from build123d import *

# Parameters (mm, degrees)
F1_DEPTH = 25
F2_R     = 1.5
F3_DEPTH = 1.5
F4_R     = 1.5
F5_DEPTH = 1.5


with BuildPart() as f1:
    # F0 (on Right) → F1 (new body, symmetric)
    with BuildSketch(Plane.YZ):
        Polygon((-9.6592582629, -7.411809549), (-8.1592582629, -7.411809549), (-8.1592582629, 10.6333523918), (9.2710296952, 5.9629208095), (9.6592582629, 7.411809549), (-9.6592582629, 12.588190451), align=None)
    extrude(amount=F1_DEPTH, both=True)

    # F2 (on face) → F3 (cut, through all)
    with BuildSketch(Plane.XZ.offset(9.6592582629)):
        Circle(F2_R)
    extrude(amount=-F3_DEPTH, mode=Mode.SUBTRACT)

    # F4 (on face) → F5 (cut, through all)
    with BuildSketch(Plane(origin=(0, 2.5, 9.3301270189), x_dir=(1, 0, 0), z_dir=(0, 0.2588190451, 0.9659258263))):
        with Locations((0, 3.411809549)):
            Circle(F4_R)
    extrude(amount=-F5_DEPTH, mode=Mode.SUBTRACT)


solid = f1.part
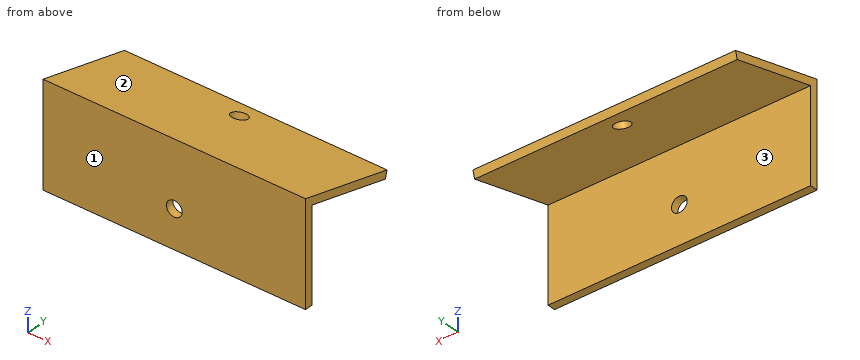
Geometry check sheet. Reference: the model listing, model coordinates, mm. Face numbers are marked on the shaded views. Coordinates: 2 decimals unless noted, no trailing zeros. Order: outer loops, then holes, each group sorted by start corner. A loop starts at its lowest first (then second) coordinate and runs counter-clockwise, first axis right, second up. Notation, with made-up numbers: (15, -3.75) - (34, -3.75) arc R36 cw to (34, 34.25) - close; hole circle Ø10 at (78, 33.25). An arc over 180 degrees is marked (long way). Answer in a Markdown table with one row per item. Add a question column.
1) Cross-section at A-A, the plane z = 0. Record the cut outline in (x, y).
2) Release check for a two-part mould opening along Y. For the marked faces 1, 2 and 3 record: +Y half, -Y half, draft (parallel to the pull), parting line (faces both ways), or undercut.
3) Gauge pin test, flat ends, axial feed: P1, Ø1.5, axis at x = -19.5, z = -2.5, coming from the +Y side; P2, Ø8, axis at x = -16, z = 3.5, coming from the +Y side; P3, Ø2, axis at x = 4.5, y = 2.5, coming from the +Z side; P4, Ø5, axis at y = -7.5, z = -1.5, coming from the +X side. Record the tip position at first contact, or that the pin passes through.
4) Cross-section at D-D, the plane z = -3. Record the cut outline in (x, y), then the cut area to 3 significant figures.
5) Cross-section at C-C, the plane x = 17. Record the cut outline in (y, z), then the cut area to 3 significant figures.
6) Cross-section at B-B, the plane x = 0. Record the cut outline in (y, z), then the cut area to 3 significant figures.
7) Material ranges on line 1 along Y through (x, z) = (-14.5, 3.5); line 2 along Z through (x, y) = (0, -9); line 3 along Z through (x, y) = (0, -9.3), recorded low to high. Write a range as [from, to].
Check result:
| question | item | result |
|---|---|---|
| 1 | outline | (-25, -9.66) - (-1.5, -9.66) - (-1.5, -8.16) - (-25, -8.16) - close; (1.5, -9.66) - (25, -9.66) - (25, -8.16) - (1.5, -8.16) - close |
| 2 | face 1 | -Y half |
| 2 | face 2 | +Y half |
| 2 | face 3 | undercut |
| 3 | P1 | stops at y = -8.16 |
| 3 | P2 | stops at y = 9.66 |
| 3 | P3 | stops at z = 9.6 |
| 3 | P4 | stops at x = 25 |
| 4 | outline | (-25, -9.66) - (25, -9.66) - (25, -8.16) - (-25, -8.16) - close |
| 4 | area | 75.0 mm² |
| 5 | outline | (-9.66, -7.41) - (-8.16, -7.41) - (-8.16, 10.63) - (9.27, 5.96) - (9.66, 7.41) - (-9.66, 12.59) - close |
| 5 | area | 57.1 mm² |
| 6 | outline | (-9.66, -7.41) - (-8.16, -7.41) - (-8.16, -1.5) - (-9.66, -1.5) - close; (-9.66, 1.5) - (-8.16, 1.5) - (-8.16, 10.63) - (3.96, 7.39) - (4.35, 8.84) - (-9.66, 12.59) - close; (6.86, 6.61) - (9.27, 5.96) - (9.66, 7.41) - (7.24, 8.06) - close |
| 6 | area | 48.1 mm² |
| 7 | line 1 | y = [-9.66, -8.16] |
| 7 | line 2 | z = [-7.41, -1.5], [1.5, 12.41] |
| 7 | line 3 | z = [-7.41, -1.5], [1.5, 12.49] |
